Work out the finished part from the listing and answer in its coordinate system (mm). A direction names the side the tool comes from. Give positions to 0.01 mm unless a question says otherwise; leave off trailing zeros. Loops run counter-clockwise (first coordinate to the right, second up) from the corner with the lowest first, then second, coordinate; pieces in that order, holes last. Notation, with made-up numbers: (60.25, 69) - (107.25, 69) arc R20 cw to (107.25, 107) - close; hole circle Ø2 at (6.25, 27.5). An arc over 180 degrees is marked (long way). One line per question, with ' | ' between items.
from build123d import *

# Parameters (mm, degrees)
SKETCH1_R           = 5
BOSS_EXTRUDE1_DEPTH = 9
FILLET1_R           = 2
SKETCH2_R           = 3
CUT_EXTRUDE2_DEPTH  = 9


with BuildPart() as part:
    # Sketch1 → Boss-Extrude1 (new body)
    with BuildSketch(Plane.XY):
        with BuildLine():
            Line((-3.996251998, 18.882233703), (-3.996251998, 9.603351185))
            Line((-3.996251998, 9.603351185), (0, 9.603351185))
            Line((0, 9.603351185), (4, 9.603351185))
            Line((4, 9.603351185), (4, 18.883750084))
            ThreePointArc((4, 18.883750084), (-0.002021567, 39.425278988), (-3.996251998, 18.882233703))
        make_face()
        with Locations((0, 28.765059691)):
            Circle(SKETCH1_R, mode=Mode.SUBTRACT)
    extrude(amount=BOSS_EXTRUDE1_DEPTH)

    # Fillet1
    fillet1_edges = [part.edges().sort_by_distance(p)[0] for p in [
        (-0.002021567, 39.425278988, 9),
        (-3.996251998, 14.242792444, 9),
        (-3.996251998, 14.242792444, 0),
        (-0.002021567, 39.425278988, 0),
        (4, 14.243550634, 0),
        (4, 14.243550634, 9),
    ]]
    fillet(fillet1_edges, radius=FILLET1_R)

    # Sketch2 → Cut-Extrude2 (cut)
    with BuildSketch(Plane.XZ.offset(-9.603351185)):
        with Locations(Location((0, 4.569140721, 0), (0, 0, 270))):
            Circle(SKETCH2_R)
    extrude(amount=-CUT_EXTRUDE2_DEPTH, mode=Mode.SUBTRACT)


solid = part.part
1. Which of the six approach directions +Z, -Z, +X, -X, +Y, -Y give full straight-line access (tool end or side, diameter ignored) to faces 1 (the flat face through (0, 18.603, 5)), 2 (the flat face through (-3.996, 14, 4)), 3 (the cylindrical face through (3.43, 15.05, 8.4))?
Evaluation:
face 1: -Y | face 2: +Z, -Z, -X, -Y | face 3: +Z, +X, -Y
2. Consider L1, parallel to Y at x = 0, z = 6.5; L2, parallel to X at y = 14.25, z = 4.5; L3, parallel to X at y = 33, z = 0.75. Determine where each line is inside the solid, lowest interval first.
Evaluation:
L1: 18.6 to 23.77, 33.77 to 39.43 | L2: -4 to -3, 3 to 4 | L3: -9.3 to -2.66, 2.66 to 9.3
3. Flat-ended cylindrical pins translate along their axes: pin 1 (1.8 mm diameter, centred on x = -0.5, z = 3, fed in from -Y); pin 2 (4 mm diameter, centred on y = 14.5, z = 5.5, fed in from +X); pin 3 (2 mm diameter, centred on x = -6.5, z = 3.5, fed in from -Y). Find the tip coordinate at first contact, or state that the pin passes through.
Evaluation:
pin 1: y = 18.6 | pin 2: x = 4 | pin 3: y = 19.63
4. Determine the mould class of faces 4 (the cylindrical face through (0.409, 39.417, 4.465)), 5 (the cylindrical face through (-3.426, 14.896, 0.601)), 6 (the cylindrical face through (-1.084, 23.884, 4.437)) for opening direction X: +X half, -X half, draft (parallel to the pull), parting line (faces both ways), or undercut.
Evaluation:
face 4: parting line | face 5: -X half | face 6: undercut
5. Find section C-C on z = 0.75. Write down the section's boundary in (x, y).
Evaluation:
outline: (-3.56, 9.6) - (3.56, 9.6) - (3.56, 19.18) arc R10.22 ccw (long way) to (-3.56, 19.18) - close; hole circle Ø10 at (0, 28.77)
6. Find section A-A on y = 17.5. Write down the section's boundary in (x, z), then the cut area to 3 significant figures.
Evaluation:
outline: (-4, 2) arc R2 ccw to (-2, 0) - (2, 0) arc R2 ccw to (4, 2) - (4, 7) arc R2 ccw to (2, 9) - (-2, 9) arc R2 ccw to (-4, 7) - close; hole circle Ø6 at (0, 4.57) | area: 40.3 mm2
7. Find section B-B on z = 6.5. Write down the section's boundary in (x, y).
Evaluation:
outline: (-4, 9.6) - (-2.3, 9.6) - (-2.3, 18.6) - (2.3, 18.6) - (2.3, 9.6) - (4, 9.6) - (4, 18.88) arc R10.66 ccw (long way) to (-4, 18.88) - close; hole circle Ø10 at (0, 28.77)
